Could you check a few things on this drawing? It's one solid part, dimensions in mm from its lowest x, y, z. Give positions to 0.01 mm unless a question says otherwise; leave off trailing zeros. Order: outer loops, then holes, each group sorted by start corner. A loop starts at its lowest first (then second) coordinate and runs counter-clockwise, first axis right, second up. Notation, with made-up numbers: (12.25, 10) -> (70.25, 10) arc R23 cw to (70.25, 47) -> close; hole circle Ø5 at (-38.75, 76.25). An arc over 180 degrees is marked (long way). Write each question's results on one line, items separated by ' | '. Start each with the question number.
Q1. Imagine slicing it at D-D, the plane z = 23. Please give me the cut outline in (x, y).
Q2. Thinking about a two-plate mould opening in Z: for the marked faces 1, 2 and 3, which applies, pulls with the +Z half, pulls with the -Z half, needs draft (parallel to the pull), parting line crosses it, or undercut?
Q3. I'm going to push flat-ended pins straight in: pin 1 (3.5 mm diameter, centred on x = 10, z = 37, fed in from -Y); pin 2 (1.5 mm diameter, centred on y = 1.5, z = 6.5, fed in from +X); pin 3 (2.5 mm diameter, centred on x = 3, z = 30, fed in from +Y); pin 4 (1.5 mm diameter, centred on y = 2.5, z = 16, fed in from -X). Where does each tip first touch, or does it pass through?
Q4. Imagine slicing it at A-A, the plane z = 30. Please give me the cut outline in (x, y).
Q5. Imagine slicing it at B-B, the plane x = 17. Please give me the cut outline in (y, z).
Q6. Imagine slicing it at C-C, the plane y = 1.55. Please give me the cut outline in (x, z).
Q7. I need wall thicknesses on line 1 along X through (y, z) = (2.5, 29.5); line 2 along X through (y, z) = (1.05, 36.5); line 3 along X through (y, z) = (1.9, 7.5). Which ranges of each line are inside material? Lowest first, please. Write a range as [from, to].
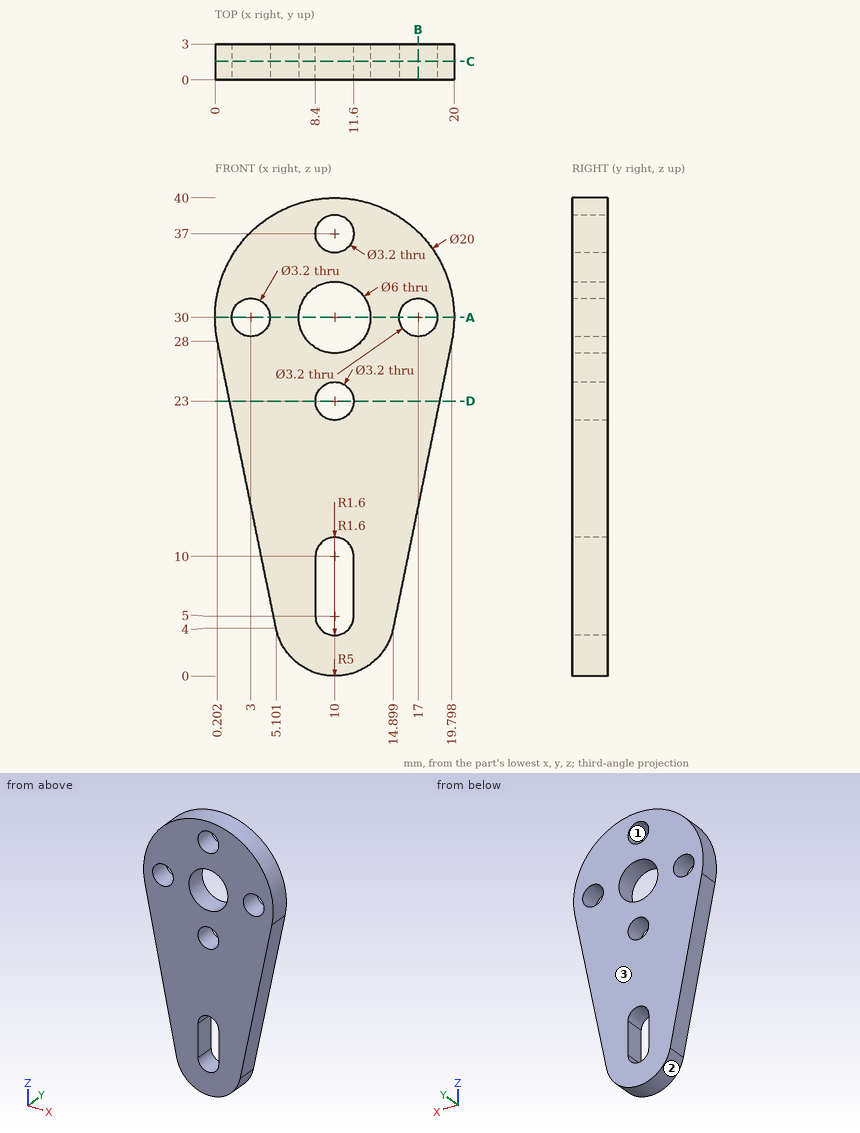
Geometry check:
1) outline: (1.22, 0) -> (8.4, 0) -> (8.4, 3) -> (1.22, 3) -> close; (11.6, 0) -> (18.78, 0) -> (18.78, 3) -> (11.6, 3) -> close
2) face 1: undercut | face 2: pulls with the -Z half | face 3: needs draft
3) pin 1: y = 0 | pin 2: x = 15.56 | pin 3: through | pin 4: x = 2.5
4) outline: (0, 0) -> (1.4, 0) -> (1.4, 3) -> (0, 3) -> close; (4.6, 0) -> (7, 0) -> (7, 3) -> (4.6, 3) -> close; (13, 0) -> (15.4, 0) -> (15.4, 3) -> (13, 3) -> close; (18.6, 0) -> (20, 0) -> (20, 3) -> (18.6, 3) -> close
5) outline: (0, 14.29) -> (3, 14.29) -> (3, 28.4) -> (0, 28.4) -> close; (0, 31.6) -> (3, 31.6) -> (3, 37.14) -> (0, 37.14) -> close
6) outline: (0.2, 28) -> (5.1, 4) arc R5 ccw to (14.9, 4) -> (19.8, 28) arc R10 ccw (long way) to start; hole circle Ø3.2 at (3, 30); hole circle Ø6 at (10, 30); hole (8.4, 5) arc R1.6 ccw to (11.6, 5) -> (11.6, 10) arc R1.6 ccw to (8.4, 10) -> close; hole circle Ø3.2 at (10, 23); hole circle Ø3.2 at (10, 37); hole circle Ø3.2 at (17, 30)
7) line 1: [0.01, 1.48], [4.52, 7.04], [12.96, 15.48], [18.52, 19.99] | line 2: [2.4, 8.48], [11.52, 17.6] | line 3: [4.39, 8.4], [11.6, 15.61]
